Model file for the job. Use its own axes, mm. Round coordinates to 2 decimals unless told otherwise and drop trailing zeros. Order: outer loops, then holes, each group sorted by start corner. A loop starts at its lowest first (then second) coordinate and runs counter-clockwise, first axis right, second up. Notation, with made-up numbers: (87, -10) - (128, -10) arc R28 cw to (128, 19) - close; hole circle Ø4 at (-25.5, 89). An arc over 180 degrees is marked (long way). Answer as CSV lines item,"result". Start each with the question number.
1. Band-saw the part on A-A on z = -450. List the corners of the cut face in (x, y), then the cut area to 3 significant figures.
2. Pin check, flat tips, straight feed: pin 1 Ø11.5 at (y, z) = (-232.5, -403) entering from -X; pin 2 Ø19 at (x, z) = (523.5, -267.5) entering from +Y; pin 3 Ø2 at (x, y) = (-387.5, -159) entering from -Z. Stop position of each tip, or through.
3. Wall check: line 1 along Y through (x, z) = (516.5, -325); line 2 along X through (y, z) = (242, -450.5); line 3 along Z through (x, y) = (-168.5, 193). Give the ranges that are in metal, low to high. Write a range as [from, to].
4. Band-saw the part on C-C on x = -255.5. List the corners of the cut face in (y, z), then the cut area to 3 significant figures.
5. Band-saw the part on D-D on y = 43. List the corners of the cut face in (x, z).
6. Band-saw the part on B-B on y = -235.5. List the corners of the cut face in (x, z), then the cut area to 3 significant figures.
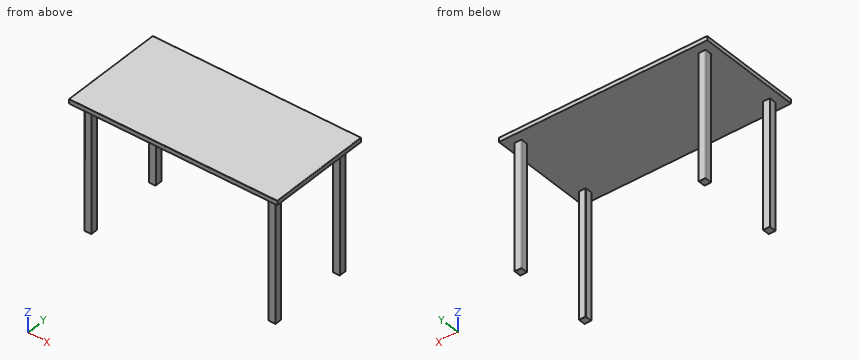
```python
from build123d import *

# Parameters (mm, degrees)
SKETCH1_W           = 1200
SKETCH1_H           = 600
BOSS_EXTRUDE1_DEPTH = 25
SKETCH2_W           = 40
SKETCH2_H           = 40
BOSS_EXTRUDE2_DEPTH = 750
FILLET1_R           = 2


with BuildPart() as part:
    # Sketch1 → Boss-Extrude1 (new body)
    with BuildSketch(Plane.XY):
        Rectangle(SKETCH1_W, SKETCH1_H)
    extrude(amount=BOSS_EXTRUDE1_DEPTH)

    # Sketch2 → Boss-Extrude2 (add)
    with BuildSketch(Plane.XY.offset(25)):
        with Locations((-530, -230)):
            Rectangle(SKETCH2_W, SKETCH2_H)
        with Locations((530, -230)):
            Rectangle(SKETCH2_W, SKETCH2_H)
        with Locations((-530, 230)):
            Rectangle(SKETCH2_W, SKETCH2_H)
        with Locations((530, 230)):
            Rectangle(SKETCH2_W, SKETCH2_H)
    extrude(amount=-BOSS_EXTRUDE2_DEPTH)

    # Fillet1
    fillet1_edges = [part.edges().sort_by_distance(p)[0] for p in [
        (510, 250, -362.5),
        (550, 230, -725),
        (510, 210, -362.5),
        (530, 250, -725),
        (-550, 250, -362.5),
        (-510, 230, -725),
        (-550, 210, -362.5),
        (-530, 250, -725),
        (510, -210, -362.5),
        (550, -230, -725),
        (530, -250, -725),
        (530, -210, -725),
        (-550, -230, -725),
        (-510, -230, -725),
        (-550, -250, -362.5),
        (-530, -210, -725),
        (-600, 0, 25),
        (600, 0, 25),
        (0, -300, 25),
        (0, 300, 25),
    ]]
    fillet(fillet1_edges, radius=FILLET1_R)


solid = part.part
```
Reply:
1,outline,"(-550, -248) arc R2 ccw to (-548, -250) - (-510, -250) - (-510, -210) - (-550, -210) - close; (-550, 212) arc R2 ccw to (-548, 210) - (-510, 210) - (-510, 250) - (-548, 250) arc R2 ccw to (-550, 248) - close; (510, -250) - (550, -250) - (550, -210) - (512, -210) arc R2 ccw to (510, -212) - close; (510, 212) arc R2 ccw to (512, 210) - (550, 210) - (550, 250) - (512, 250) arc R2 ccw to (510, 248) - close"
1,area,"6,390 mm2"
2,pin 1,"stops at x = -550"
2,pin 2,"stops at y = 250"
2,pin 3,"stops at z = 0"
3,line 1,"y = [-250, -210], [210, 250]"
3,line 2,"x = [-550, -510], [510, 550]"
3,line 3,"z = [0, 25]"
4,outline,"(-300, 0) - (300, 0) - (300, 23) arc R2 ccw to (298, 25) - (-298, 25) arc R2 ccw to (-300, 23) - close"
4,area,"15,000 mm2"
5,outline,"(-600, 0) - (600, 0) - (600, 23) arc R2 ccw to (598, 25) - (-598, 25) arc R2 ccw to (-600, 23) - close"
6,outline,"(-600, 0) - (-550, 0) - (-550, -723) arc R2 ccw to (-548, -725) - (-512, -725) arc R2 ccw to (-510, -723) - (-510, 0) - (510, 0) - (510, -725) - (548, -725) arc R2 ccw to (550, -723) - (550, 0) - (600, 0) - (600, 23) arc R2 ccw to (598, 25) - (-598, 25) arc R2 ccw to (-600, 23) - close"
6,area,"88,000 mm2"
